from build123d import *

# Parameters (mm, degrees)
SKETCH1_W           = 60
SKETCH1_H           = 5
SKETCH1_R           = 10
SKETCH1_R_2         = 5
BOSS_EXTRUDE1_DEPTH = 5
SKETCH2_R           = 3.25
BOSS_EXTRUDE2_DEPTH = 10
FILLET1_R           = 1


with BuildPart() as part:
    # Sketch1 → Boss-Extrude1 (new, symmetric)
    with BuildSketch(Plane.XY):
        with BuildLine():
            Line((-50, 80.817230765), (-50, 0))
            ThreePointArc((-50, 0), (-40, 10), (-30, 0))
            Line((-30, 0), (-30, 75.817230765))
            Line((-30, 75.817230765), (-30, 80.817230765))
            Line((-30, 80.817230765), (-50, 80.817230765))
        make_face()
        with Locations((0, 78.317230765)):
            Rectangle(SKETCH1_W, SKETCH1_H)
        with BuildLine():
            Line((50, 80.817230765), (30, 80.817230765))
            Line((30, 80.817230765), (30, 75.817230765))
            Line((30, 75.817230765), (30, 0))
            ThreePointArc((30, 0), (40, 10), (50, 0))
            Line((50, 0), (50, 80.817230765))
        make_face()
        with Locations((-40, 0)):
            Circle(SKETCH1_R)
        with Locations((-40, 0)):
            Circle(SKETCH1_R_2, mode=Mode.SUBTRACT)
        with Locations((40, 0)):
            Circle(SKETCH1_R)
        with Locations((40, 0)):
            Circle(SKETCH1_R_2, mode=Mode.SUBTRACT)
    extrude(amount=BOSS_EXTRUDE1_DEPTH, both=True)

    # Sketch2 → Boss-Extrude2 (add)
    with BuildSketch(Plane.XY.offset(5)):
        with BuildLine():
            Line((-5, 75.817230765), (-5, 68.317230765))
            ThreePointArc((-5, 68.317230765), (0, 63.317230765), (5, 68.317230765))
            Line((5, 68.317230765), (5, 75.817230765))
            Line((5, 75.817230765), (-5, 75.817230765))
        make_face()
        with Locations((0, 68.317230765)):
            Circle(SKETCH2_R, mode=Mode.SUBTRACT)
    extrude(amount=-BOSS_EXTRUDE2_DEPTH)

    # Fillet1
    fillet1_edges = [part.edges().sort_by_distance(p)[0] for p in [
        (-50, 80.817230765, 0),
        (50, 80.817230765, 0),
        (30, 75.817230765, 0),
        (-30, 75.817230765, 0),
        (-5, 75.817230765, 0),
        (5, 75.817230765, 0),
    ]]
    fillet(fillet1_edges, radius=FILLET1_R)


solid = part.part
Input: part model. Units: mm. Frame: model coordinates. A direction names the side the tool comes from. Give positions to 0.01 mm unless a question says otherwise; leave off trailing zeros. Order: outer loops, then holes, each group sorted by start corner. A loop starts at its lowest first (then second) coordinate and runs counter-clockwise, first axis right, second up. Notation, with made-up numbers: (45, 84.25) - (55, 84.25) arc R17 cw to (55, 101.25) - close; hole circle Ø1 at (-16, -4). An arc over 180 degrees is marked (long way). Answer as a JSON object with one key per item and string values. Group by question number.
Q1. Cut plane A-A, the plane x = 0. Output: boundary loops of the cut face in (y, z).
Q2. Mould query, pull axis Y, two halves, no side actions, for faces 3 (the face through (1, 80.817, 0)), 4 (the face through (-0.705, 65.145, 0.07)), 5 (the face through (40, -10, 0)). Classes: pulls with the +Y half, pulls with the -Y half, needs draft (parallel to the pull), parting line crosses it, or undercut.
Q3. First-contact query: pin 1 Ø7.5 at (x, y) = (0, 68.32) entering from -Z; pin 2 Ø6 at (x, y) = (-40, 0) entering from +Z; pin 3 Ø5 at (x, z) = (-19, 0) entering from -Y. Flat tips, straight axial feed; report the tip coordinate or a pass-through.
Q4. Cut plane C-C, the plane z = 1.5. Output: boundary loops of the cut face in (x, y), then the cut area to 3 significant figures.
Q5. Line query: probe 1 along Y at (x, z) = (0, -0.5); probe 2 along X at (y, z) = (49, -1.25); probe 3 along Y at (x, z) = (-40.5, -3.25). Output: solid intervals per line, ascending.
Q6. Set-up query: faces 1 (the face through (-18, 75.817, 0)), 2 (the face through (-50, 40, 0)). Return all of +Z, -Z, +X, -X, +Y, -Y with unobstructed straight access to the full face (end or side cutting, diameter ignored); none if empty.
Q7. Cut plane B-B, the plane y = 35. Output: boundary loops of the cut face in (x, z), then the cut area to 3 significant figures.
Results:
{
 "1": {"outline": "(63.32, -5) - (65.07, -5) - (65.07, 5) - (63.32, 5) - close; (71.57, -5) - (80.82, -5) - (80.82, 5) - (71.57, 5) - close"},
 "2": {"face 3": "pulls with the +Y half", "face 4": "undercut", "face 5": "pulls with the -Y half"},
 "3": {"pin 1": "z = -5", "pin 2": "through", "pin 3": "y = 75.82"},
 "4": {"outline": "(-50, 0) arc R10 ccw to (-30, 0) - (-30, 74.82) arc R1 cw to (-29, 75.82) - (-6, 75.82) arc R1 cw to (-5, 74.82) - (-5, 68.32) arc R5 ccw to (5, 68.32) - (5, 74.82) arc R1 cw to (6, 75.82) - (29, 75.82) arc R1 cw to (30, 74.82) - (30, 0) arc R10 ccw to (50, 0) - (50, 79.82) arc R1 ccw to (49, 80.82) - (-49, 80.82) arc R1 ccw to (-50, 79.82) - close; hole circle Ø10 at (-40, 0); hole circle Ø6.5 at (0, 68.32); hole circle Ø10 at (40, 0)", "area": "3,770 mm^2"},
 "5": {"probe 1": "63.32 to 65.07, 71.57 to 80.82", "probe 2": "-50 to -30, 30 to 50", "probe 3": "-9.99 to -4.97, 4.97 to 80.82"},
 "6": {"face 1": "+Z, -Z, -Y", "face 2": "+Z, -Z, -X, +Y, -Y"},
 "7": {"outline": "(-50, -5) - (-30, -5) - (-30, 5) - (-50, 5) - close; (30, -5) - (50, -5) - (50, 5) - (30, 5) - close", "area": "400 mm^2"}
}
